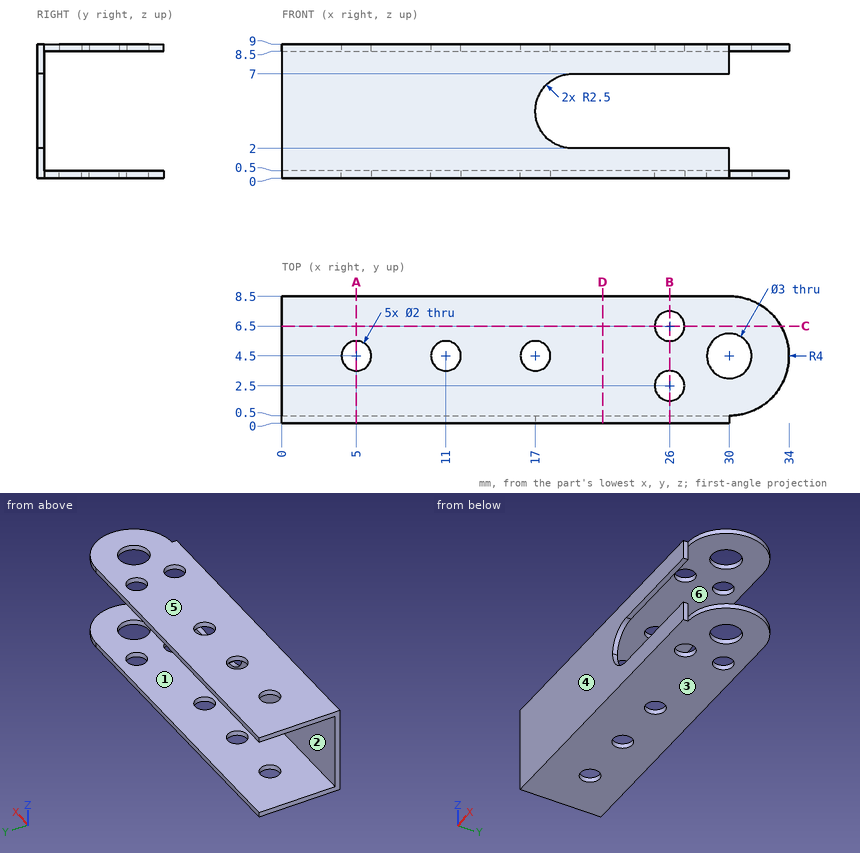
Job drawing, mm, ordinate dimensions from the low corner. One solid piece. A direction names the side the tool comes from. Coordinates: 2 decimals unless noted, no trailing zeros. Order: outer loops, then holes, each group sorted by start corner. A loop starts at its lowest first (then second) coordinate and runs counter-clockwise, first axis right, second up. Notation, with made-up numbers: (18, -35.75) -> (29, -35.75) arc R28 cw to (29, -17.75) -> close; hole circle Ø9 at (-37.75, 72.5). An arc over 180 degrees is marked (long way). Return JSON: item names as keys, results as strings. Group by question number.
Item 1: Tool access for the marked faces 5 and 6: list every direction of +Z, -Z, +X, -X, +Y, -Y with a clear straight run to the whole face (end or side of a thin tool).
Item 2: Wall check: line 1 along Y through (x, z) = (26, 0.2); line 2 along Z through (x, y) = (8.5, 2.5); line 3 along Y through (x, z) = (11, 8.65). Give the ranges that are in metal, low to high. Write a range as [from, to].
Item 3: Flat gauge pins, fed straight in: P1, Ø3, axis at x = 14, z = 2.5, coming from the +Y side; P2, Ø5, axis at y = 7.5, z = 1.5, coming from the +X side; P3, Ø0.6, axis at y = 0.5, z = 8, coming from the +X side. Where does each tip first touch, or does it go through?
Item 4: Saw through at A-A on x = 5. Write the cut outline in (y, z).
Item 5: Pull direction Z, two halves, no side cores. Call the marked faces 1, 2, 3 and 4: pulls with the +Z half, pulls with the -Z half, needs draft (parallel to the pull), parting line crosses it, or undercut.
Item 6: Saw through at C-C on y = 6.5. Write the cut outline in (x, z).
Item 7: Saw through at D-D on x = 21.5. Write the cut outline in (y, z).
Item 8: Saw through at B-B on x = 26. Write the cut outline in (y, z).
Values found:
{
 "1": {"face 5": "+Z, +X, -X, +Y, -Y", "face 6": "+X, -X, +Y"},
 "2": {"line 1": "y = [0, 1.5], [3.5, 5.5], [7.5, 8.5]", "line 2": "z = [0, 0.5], [8.5, 9]", "line 3": "y = [0, 3.5], [5.5, 8.5]"},
 "3": {"P1": "stops at y = 0.5", "P2": "stops at x = 33.94", "P3": "stops at x = 30"},
 "4": {"outline": "(0, 0) -> (3.5, 0) -> (3.5, 0.5) -> (0.5, 0.5) -> (0.5, 8.5) -> (3.5, 8.5) -> (3.5, 9) -> (0, 9) -> close; (5.5, 0) -> (8.5, 0) -> (8.5, 0.5) -> (5.5, 0.5) -> close; (5.5, 8.5) -> (8.5, 8.5) -> (8.5, 9) -> (5.5, 9) -> close"},
 "5": {"face 1": "undercut", "face 2": "undercut", "face 3": "pulls with the -Z half", "face 4": "needs draft"},
 "6": {"outline": "(0, 0) -> (25, 0) -> (25, 0.5) -> (0, 0.5) -> close; (0, 8.5) -> (25, 8.5) -> (25, 9) -> (0, 9) -> close; (27, 0) -> (33.46, 0) -> (33.46, 0.5) -> (27, 0.5) -> close; (27, 8.5) -> (33.46, 8.5) -> (33.46, 9) -> (27, 9) -> close"},
 "7": {"outline": "(0, 0) -> (8.5, 0) -> (8.5, 0.5) -> (0.5, 0.5) -> (0.5, 2) -> (0, 2) -> close; (0, 7) -> (0.5, 7) -> (0.5, 8.5) -> (8.5, 8.5) -> (8.5, 9) -> (0, 9) -> close"},
 "8": {"outline": "(0, 0) -> (1.5, 0) -> (1.5, 0.5) -> (0.5, 0.5) -> (0.5, 2) -> (0, 2) -> close; (0, 7) -> (0.5, 7) -> (0.5, 8.5) -> (1.5, 8.5) -> (1.5, 9) -> (0, 9) -> close; (3.5, 0) -> (5.5, 0) -> (5.5, 0.5) -> (3.5, 0.5) -> close; (3.5, 8.5) -> (5.5, 8.5) -> (5.5, 9) -> (3.5, 9) -> close; (7.5, 0) -> (8.5, 0) -> (8.5, 0.5) -> (7.5, 0.5) -> close; (7.5, 8.5) -> (8.5, 8.5) -> (8.5, 9) -> (7.5, 9) -> close"}
}
